Model file for the job. Use its own axes, mm. Face numbers are marked on the shaded views. A direction names the side the tool comes from. Round coordinates to 2 decimals unless told otherwise and drop trailing zeros. Loops run counter-clockwise (first coordinate to the right, second up) from the corner with the lowest first, then second, coordinate; pieces in that order, holes last. Notation, with made-up numbers: M -36.75,79.25 L -11.75,79.25 A25 cw -11.75,91.25 Z; hole C 54,46.25 d2. An arc over 180 degrees is marked long. Use a Markdown table: item, result. Add a question column.
Q1. Cut at B-B (z = 70.75). Give the cut face in (x, y), plus the area to 3 significant figures.
Q2. Tool access for the marked faces 1, 2 and 3: list every direction of +Z, -Z, +X, -X, +Y, -Y with a clear straight run to the whole face (end or side of a thin tool).
Q3. Probe line 1 (Z direction, x = 14, y = 0); line 2 (Z direction, x = 6, y = 1); line 3 (Y direction, x = 13.25, z = 74.2). List the from-to ranges inside material, lowest first. Write a range as from..to.
Q4. Cut at A-A (x = 0). Give the cut face in (y, z).
Q5. Cut at C-C (x = 13.5). Give the cut face in (y, z), plus the area to 3 significant figures.
Q6. Cut at D-D (z = 74.2). Give the cut face in (x, y).
Q7. Pin check, flat tips, straight feed: pin 1 (12 mm diameter, centred on x = 4.5, z = 63, fed in from -Y); pin 2 (1.1 mm diameter, centred on y = 0, z = 51, fed in from +X); pin 3 (2 mm diameter, centred on x = 14.5, z = 69.5, fed in from -Y); pin 4 (1.5 mm diameter, centred on x = -1, z = 50.5, fed in from -Y). Stop position of each tip, or through.
from build123d import *

# Parameters (mm, degrees)
CYLINDER060_R     = 1.2
CYLINDER060_DEPTH = 10
ARRAY013_COUNT    = 3
CYLINDER061_R     = 4
CYLINDER061_DEPTH = 20
BOX014_W          = 8
BOX014_H          = 1
BOX014_DEPTH      = 3
CYLINDER059_R     = 20.2
CYLINDER059_DEPTH = 5


with BuildPart() as pos_plate_screws:
    # Cylinder060 → Cylinder060 (new body)
    with BuildSketch(Plane(origin=(10.5, 0, 74.2), x_dir=(0, 0, -1), z_dir=(1, 0, 0))):
        Circle(CYLINDER060_R)
    extrude(amount=CYLINDER060_DEPTH)

    # Array013: pos-plate-screws ×3 about axis
    array013_axis = Axis((0, 0, 0), (0, 0, 1))


with BuildPart() as pos_plate_screws_1:
    add(pos_plate_screws.part)
    for i in range(1, ARRAY013_COUNT):
        add(pos_plate_screws.part.rotate(array013_axis, i * 360 / ARRAY013_COUNT))


with BuildPart() as pos_cylinder:
    # Cylinder061 → Cylinder061 (new body)
    with BuildSketch(Plane.XY.offset(51.7)):
        Circle(CYLINDER061_R)
    extrude(amount=CYLINDER061_DEPTH)


with BuildPart() as pos_pick:
    # Box014 → Box014 (new body)
    with BuildSketch(Plane(origin=(-4, -0.5, 48.7), x_dir=(1, 0, 0), z_dir=(0, 0, 1))):
        with Locations((4, 0.5)):
            Rectangle(BOX014_W, BOX014_H)
    extrude(amount=BOX014_DEPTH)


with BuildPart() as turret_pos_pick:
    # Cylinder059 → Cylinder059 (new body)
    with BuildSketch(Plane.XY.offset(71.7)):
        Circle(CYLINDER059_R)
    extrude(amount=CYLINDER059_DEPTH)

    # Fusion026: union pos-cylinder, pos-pick
    add(pos_cylinder.part)
    add(pos_pick.part)

    # Cut048: cut pos-plate-screws
    add(pos_plate_screws_1.part, mode=Mode.SUBTRACT)


solid = turret_pos_pick.part
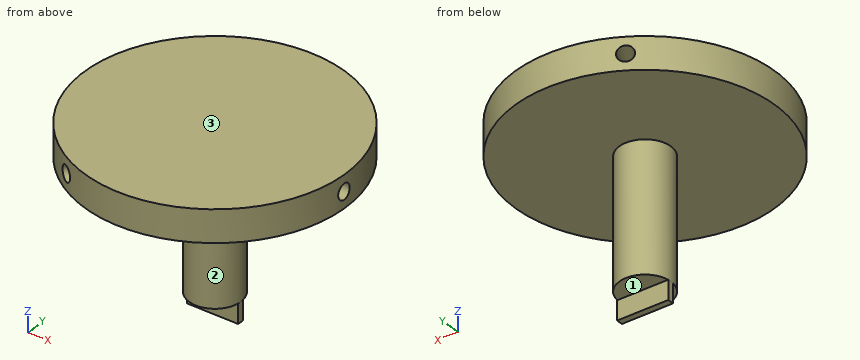
Checked values:
| question | item | result |
|---|---|---|
| 1 | outline | C 0,0 d8 |
| 1 | area | 50.3 mm^2 |
| 2 | face 1 | -Z, +X, -X, +Y |
| 2 | face 2 | -Z |
| 2 | face 3 | +Z, +X, -X, +Y, -Y |
| 3 | line 1 | z = 71.7..73, 75.4..76.7 |
| 3 | line 2 | z = 71.7..76.7 |
| 3 | line 3 | y = -15.25..-1.2, 1.2..15.25 |
| 4 | outline | M -20.2,71.7 L -4,71.7 L -4,51.7 L -0.5,51.7 L -0.5,48.7 L 0.5,48.7 L 0.5,51.7 L 4,51.7 L 4,71.7 L 20.2,71.7 L 20.2,76.7 L -20.2,76.7 Z |
| 5 | outline | M -15.03,71.7 L 15.03,71.7 L 15.03,76.7 L -15.03,76.7 Z; hole C 0,74.2 d2.4 |
| 5 | area | 146 mm^2 |
| 6 | outline | M -11.12,-16.86 L -6.29,-8.49 L -4.21,-9.69 L -9.04,-18.06 A20.2 ccw 20.16,-1.2 L 10.5,-1.2 L 10.5,1.2 L 20.16,1.2 A20.2 ccw -9.04,18.06 L -4.21,9.69 L -6.29,8.49 L -11.12,16.86 A20.2 ccw Z |
| 7 | pin 1 | stops at y = -4 |
| 7 | pin 2 | stops at x = 4 |
| 7 | pin 3 | passes through |
| 7 | pin 4 | stops at y = -0.5 |
